Read the model definition and answer for the solid it produces. Units are mm, in the model's axes. A direction names the side the tool comes from. Give positions to 0.01 mm unless a question says otherwise; leave off trailing zeros. Write each loop counter-clockwise with the first axis right and the second up, starting at its lowest first coordinate (ties: lowest second). Pieces come first, ordered by that corner, then holes.
Autodesk Fusion 360 part; units mm, degrees
sketch "Sketch1" plane through (0, 0, 0) normal (0, 0, 1) x (1, 0, 0)
  line L0 (140, -145) -> (-140, -145)
  line L1 (-140, -145) -> (-140, 145)
  line L2 (-140, 145) -> (140, 145)
  line L3 (140, 145) -> (140, -145)
  line L4 (140, -145) -> (-140, 145) construction
  line L5 (-140, -145) -> (140, 145) construction
  dimension "d1" = 280
  dimension "d2" = 290
extrude "Extrude1" add sketch "Sketch1" along normal blind 350
sketch "Sketch2" plane through (0, -145, 0) normal (0, -1, 0) x (1, 0, 0)
  line L0 (-140, 0) -> (140, 0)
  line L1 (140, 0) -> (140, 350)
  line L2 (140, 350) -> (-140, 350)
  line L3 (-140, 350) -> (-140, 0)
  line L4 (25, 125) -> (-125, 125)
  line L5 (-125, 125) -> (-125, 325)
  line L6 (-125, 325) -> (25, 325)
  line L7 (25, 325) -> (25, 125)
  line L8 (25, 125) -> (-125, 325) construction
  line L9 (-125, 125) -> (25, 325) construction
  point P0 (-50, 225)
extrude "Extrude2" cut sketch "Sketch2" against normal blind 200 contours L4 L5 L6 L7
sketch "Sketch3" plane through (0, -145, 0) normal (0, -1, 0) x (1, 0, 0)
  line L0 (-125, 125) -> (-125, 325)
  line L1 (-125, 325) -> (25, 325)
  line L2 (25, 325) -> (25, 125)
  line L3 (25, 125) -> (-125, 125)
  line L4 (-140, 0) -> (140, 0)
  line L5 (140, 0) -> (140, 350)
  line L6 (140, 350) -> (-140, 350)
  line L7 (-140, 350) -> (-140, 0)
  line L8 (123.6698, 300.3073) -> (46.6698, 300.3073)
  line L9 (46.6698, 300.3073) -> (46.6698, 325.3073)
  line L10 (46.6698, 325.3073) -> (123.6698, 325.3073)
  line L11 (123.6698, 325.3073) -> (123.6698, 300.3073)
  line L12 (123.6698, 300.3073) -> (46.6698, 325.3073) construction
  line L13 (46.6698, 300.3073) -> (123.6698, 325.3073) construction
  circle A0 centre (70, 260) radius 9
  circle A1 centre (100, 260) radius 9
  circle A2 centre (70, 230) radius 9
  circle A3 centre (100, 230) radius 9
  line L14 (25, 22.9549) -> (-125, 22.9549)
  line L15 (-125, 22.9549) -> (-125, 112.9549)
  line L16 (-125, 112.9549) -> (25, 112.9549)
  line L17 (25, 112.9549) -> (25, 22.9549)
  line L18 (25, 22.9549) -> (-125, 112.9549) construction
  line L19 (-125, 22.9549) -> (25, 112.9549) construction
  line L20 (85, 185) -> (95, 185)
  line L21 (95, 185) -> (95, 160)
  line L22 (95, 160) -> (85, 160)
  line L23 (85, 160) -> (85, 185)
  point P0 (85.1698, 312.8073)
  point P1 (-50, 67.9549)
  dimension "d7" = 77
  dimension "d8" = 25
  dimension "d9" = 18
  dimension "d10" = 18
  dimension "d11" = 18
  dimension "d12" = 18
  dimension "d13" = 150
  dimension "d14" = 90
extrude "Extrude3" add sketch "Sketch3" along normal blind 2 contours L8 L9 L10 L11
sketch "Sketch4" plane through (0, 55, 0) normal (0, -1, 0) x (1, 0, 0)
  line L0 (25, 325) -> (-125, 325)
  line L1 (-125, 325) -> (-125, 125)
  line L2 (-125, 125) -> (25, 125)
  line L3 (25, 125) -> (25, 325)
  line L4 (-125, 200.3816) -> (25, 200.3816)
  line L5 (25, 200.3816) -> (25, 195.3816)
  line L6 (25, 195.3816) -> (-125, 195.3816)
  line L7 (-125, 195.3816) -> (-125, 200.3816)
  line L8 (-125, 261.7004) -> (25, 261.7004)
  line L9 (25, 261.7004) -> (25, 256.7004)
  line L10 (25, 256.7004) -> (-125, 256.7004)
  line L11 (-125, 256.7004) -> (-125, 261.7004)
  dimension "d17" = 5
  dimension "d18" = 150
  dimension "d19" = 5
extrude "Extrude4" add sketch "Sketch4" along normal blind 150 contours L1 L3 L8 L9 L10 L11 | L1 L3 L4 L5 L6 L7
sketch "Sketch5" plane through (0, 0, 125) normal (0, 0, 1) x (-1, 0, 0)
  line L0 (125, 145) -> (-25, 145)
  line L1 (-25, 145) -> (-25, -55)
  line L2 (-25, -55) -> (125, -55)
  line L3 (125, -55) -> (125, 145)
  line L4 (-25, 135) -> (125, 135)
  line L5 (125, 135) -> (125, 5)
  line L6 (125, 5) -> (-25, 5)
  line L7 (-25, 5) -> (-25, 135)
  line L8 (-25, 135) -> (125, 5) construction
  line L9 (125, 135) -> (-25, 5) construction
  point P0 (50, 70)
  dimension "d22" = 130
extrude "Extrude5" cut sketch "Sketch5" against normal blind 75 contours L1 L3 L4 L5 L6 L7
sketch "Sketch6" plane through (0, -145, 0) normal (0, -1, 0) x (1, 0, 0)
  line L0 (123.6698, 325.3073) -> (123.6698, 300.3073)
  line L1 (123.6698, 300.3073) -> (46.6698, 300.3073)
  line L2 (46.6698, 300.3073) -> (46.6698, 325.3073)
  line L3 (46.6698, 325.3073) -> (123.6698, 325.3073)
  line L4 (-125, 125) -> (-125, 325)
  line L5 (-125, 325) -> (25, 325)
  line L6 (25, 325) -> (25, 125)
  line L7 (25, 125) -> (-125, 125)
  line L8 (-140, 0) -> (140, 0)
  line L9 (140, 0) -> (140, 350)
  line L10 (140, 350) -> (-140, 350)
  line L11 (-140, 350) -> (-140, 0)
  line L12 (25, 25) -> (-125, 25)
  line L13 (-125, 25) -> (-125, 115)
  line L14 (-125, 115) -> (25, 115)
  line L15 (25, 115) -> (25, 25)
  line L16 (25, 25) -> (-125, 115) construction
  line L17 (-125, 25) -> (25, 115) construction
  point P0 (-50, 70)
  dimension "d25" = 150
  dimension "d26" = 90
extrude "Extrude6" cut sketch "Sketch6" against normal blind 150 contours L12 L13 L14 L15
sketch "Sketch7" plane through (0, -145, 0) normal (0, -1, 0) x (1, 0, 0)
  line L0 (-125, 25) -> (-125, 115)
  line L1 (-125, 115) -> (25, 115)
  line L2 (25, 115) -> (25, 25)
  line L3 (25, 25) -> (-125, 25)
  line L4 (123.6698, 325.3073) -> (123.6698, 300.3073)
  line L5 (123.6698, 300.3073) -> (46.6698, 300.3073)
  line L6 (46.6698, 300.3073) -> (46.6698, 325.3073)
  line L7 (46.6698, 325.3073) -> (123.6698, 325.3073)
  line L8 (-125, 125) -> (-125, 325)
  line L9 (-125, 325) -> (25, 325)
  line L10 (25, 325) -> (25, 125)
  line L11 (25, 125) -> (-125, 125)
  line L12 (-140, 0) -> (140, 0)
  line L13 (140, 0) -> (140, 350)
  line L14 (140, 350) -> (-140, 350)
  line L15 (-140, 350) -> (-140, 0)
  circle A0 centre (70, 265) radius 10
  circle A1 centre (105, 265) radius 10
  circle A2 centre (70, 235) radius 10
  circle A3 centre (105, 235) radius 10
  dimension "d29" = 20
  dimension "d30" = 20
  dimension "d31" = 20
  dimension "d32" = 20
extrude "Extrude7" add sketch "Sketch7" along normal blind 3 contours A0 | A1 | A2 | A3
sketch "Sketch8" plane through (0, -145, 0) normal (0, -1, 0) x (1, 0, 0)
  circle A0 centre (105, 235) radius 10
  circle A1 centre (70, 265) radius 10
  circle A2 centre (70, 235) radius 10
  circle A3 centre (105, 265) radius 10
  line L0 (-125, 25) -> (-125, 115)
  line L1 (-125, 115) -> (25, 115)
  line L2 (25, 115) -> (25, 25)
  line L3 (25, 25) -> (-125, 25)
  line L4 (123.6698, 325.3073) -> (123.6698, 300.3073)
  line L5 (123.6698, 300.3073) -> (46.6698, 300.3073)
  line L6 (46.6698, 300.3073) -> (46.6698, 325.3073)
  line L7 (46.6698, 325.3073) -> (123.6698, 325.3073)
  line L8 (-125, 125) -> (-125, 325)
  line L9 (-125, 325) -> (25, 325)
  line L10 (25, 325) -> (25, 125)
  line L11 (25, 125) -> (-125, 125)
  line L12 (-140, 0) -> (140, 0)
  line L13 (140, 0) -> (140, 350)
  line L14 (140, 350) -> (-140, 350)
  line L15 (-140, 350) -> (-140, 0)
  line L16 (89.5, 172) -> (84.5, 172)
  line L17 (84.5, 172) -> (84.5, 198)
  line L18 (84.5, 198) -> (89.5, 198)
  line L19 (89.5, 198) -> (89.5, 172)
  line L20 (89.5, 172) -> (84.5, 198) construction
  line L21 (84.5, 172) -> (89.5, 198) construction
  point P0 (87, 185)
  dimension "d35" = 5
  dimension "d36" = 26
extrude "Extrude8" cut sketch "Sketch8" against normal blind 100 contours L16 L17 L18 L19
Item 1: Section D-D (y = -51) is taken. Write down the section's boundary in (x, z), and give its area (3 significant figures).
Result set:
outline: (-140, 0) - (140, 0) - (140, 350) - (-140, 350) - close; hole (-125, 25) - (25, 25) - (25, 195.38) - (-125, 195.38) - close; hole (-125, 200.38) - (25, 200.38) - (25, 256.7) - (-125, 256.7) - close; hole (-125, 261.7) - (25, 261.7) - (25, 325) - (-125, 325) - close; hole (84.5, 172) - (89.5, 172) - (89.5, 198) - (84.5, 198) - close
area: 54,400 mm2
Item 2: Section C-C (y = 50) is taken. Write down the section's boundary in (x, z), and give its area (3 significant figures).
Result set:
outline: (-140, 0) - (140, 0) - (140, 350) - (-140, 350) - close; hole (-125, 125) - (25, 125) - (25, 195.38) - (-125, 195.38) - close; hole (-125, 200.38) - (25, 200.38) - (25, 256.7) - (-125, 256.7) - close; hole (-125, 261.7) - (25, 261.7) - (25, 325) - (-125, 325) - close
area: 69,500 mm2
Item 3: Find the intervals of material crossed by line 1 along Z through (x, y) = (-24, -32); line 2 along Z through (x, y) = (-75.5, -128); line 3 along Z through (x, y) = (-49, 53), in increasing order.
Result set:
line 1: z = 0 to 25, 195.38 to 200.38, 256.7 to 261.7, 325 to 350
line 2: z = 0 to 25, 325 to 350
line 3: z = 0 to 125, 195.38 to 200.38, 256.7 to 261.7, 325 to 350
Item 4: Which of the six approach directions +Z, -Z, +X, -X, +Y, -Y give full straight-line access (tool end or side, diameter ignored) to faces 3 (the flat face through (-51, -19, 261.7)), 4 (the flat face through (70, -148, 235)), 5 (the flat face through (-51, -5, 120))?
Result set:
face 3: -Y
face 4: +Z, -Z, +X, -X, -Y
face 5: none
Item 5: Section A-A (x = 0.5) is taken. Write down the section's boundary in (y, z).
Result set:
outline: (-145, 0) - (145, 0) - (145, 350) - (-145, 350) - (-145, 325) - (55, 325) - (55, 261.7) - (-95, 261.7) - (-95, 256.7) - (55, 256.7) - (55, 200.38) - (-95, 200.38) - (-95, 195.38) - (55, 195.38) - (55, 125) - (-5, 125) - (-5, 115) - (5, 115) - (5, 25) - (-145, 25) - close; (-145, 115) - (-135, 115) - (-135, 125) - (-145, 125) - close
Item 6: Determine the mould class of faces 1 (the flat face through (-49, -135, 120)), 2 (the flat face through (85, -147, 313)) for opening direction X: pulls with the +X half, pulls with the -X half, needs draft (parallel to the pull), parting line crosses it, or undercut.
Result set:
face 1: undercut
face 2: needs draft
Item 7: Section B-B (z = 154) is taken. Write down the section's boundary in (x, y), and give its area (3 significant figures).
Result set:
outline: (-140, -145) - (-125, -145) - (-125, 55) - (25, 55) - (25, -145) - (140, -145) - (140, 145) - (-140, 145) - close
area: 51,200 mm2
Item 8: Each of these flat-tipped pins is pushed along its axis until it touches: pin 1 Ø0.6 at (x, y) = (84, -146) entering from +Z; pin 2 Ø1 at (x, y) = (103, -146) entering from -Z; pin 3 Ø2.5 at (x, z) = (-48.5, 198.5) entering from -Y. Where does it stop, or does it pass through?
Result set:
pin 1: stops at z = 325.31
pin 2: stops at z = 225.11
pin 3: stops at y = -95
